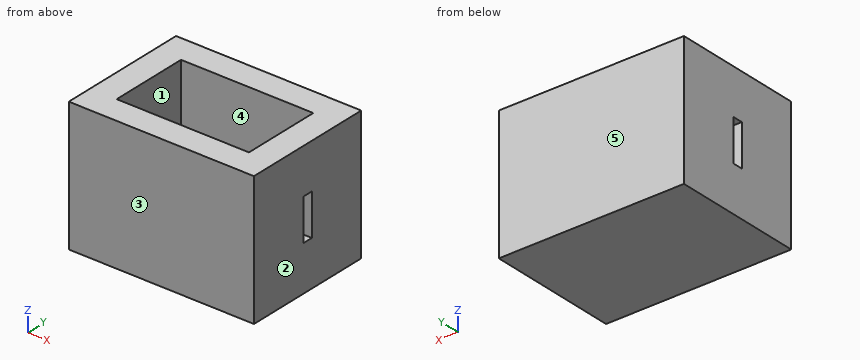
```python
from build123d import *

# Parameters (mm, degrees)
IZIM1_W                     = 12.7
IZIM1_H                     = 12.7
Y_KSEKLIK_EKSTR_ZYON1_DEPTH = 2.54
IZIM2_W                     = 4
IZIM2_H                     = 1
KES_EKSTR_ZYON1_DEPTH       = 2.54
IZIM3_W                     = 12.7
IZIM3_H                     = 12.7
Y_KSEKLIK_EKSTR_ZYON2_DEPTH = 2.54
IZIM4_W                     = 12.7
IZIM4_H                     = 12.7
Y_KSEKLIK_EKSTR_ZYON3_DEPTH = 2.54
IZIM5_W                     = 12.7
IZIM5_H                     = 7.62
Y_KSEKLIK_EKSTR_ZYON4_DEPTH = 2.54
IZIM7_W                     = 12.7
IZIM7_H                     = 12.7
Y_KSEKLIK_EKSTR_ZYON6_DEPTH = 2.54
IZIM8_W                     = 4
IZIM8_H                     = 1
KES_EKSTR_ZYON2_DEPTH       = 2.54


with BuildPart() as part:
    # Çizim1 → Yükseklik-Ekstrüzyon1 (new body)
    with BuildSketch(Plane(origin=(0, 0, 0), x_dir=(0, 0, -1), z_dir=(1, 0, 0))):
        Rectangle(IZIM1_W, IZIM1_H)
    extrude(amount=Y_KSEKLIK_EKSTR_ZYON1_DEPTH)

    # Çizim2 → Kes-Ekstrüzyon1 (cut)
    with BuildSketch(Plane(origin=(2.54, 0, 0), x_dir=(0, 0, -1), z_dir=(1, 0, 0))):
        Rectangle(IZIM2_W, IZIM2_H)
    extrude(amount=-KES_EKSTR_ZYON1_DEPTH, mode=Mode.SUBTRACT)

    # Çizim3 → Yükseklik-Ekstrüzyon2 (add)
    with BuildSketch(Plane(origin=(0, 6.35, 0), x_dir=(1, 0, 0), z_dir=(0, 1, 0))):
        with Locations((8.89, 0)):
            Rectangle(IZIM3_W, IZIM3_H)
    extrude(amount=-Y_KSEKLIK_EKSTR_ZYON2_DEPTH)

    # Çizim4 → Yükseklik-Ekstrüzyon3 (add)
    with BuildSketch(Plane.XZ.offset(6.35)):
        with Locations((8.89, 0)):
            Rectangle(IZIM4_W, IZIM4_H)
    extrude(amount=-Y_KSEKLIK_EKSTR_ZYON3_DEPTH)

    # Çizim5 → Yükseklik-Ekstrüzyon4 (add)
    with BuildSketch(Plane(origin=(0, 0, -6.35), x_dir=(-1, 0, 0), z_dir=(0, 0, -1))):
        with Locations((-8.89, 0)):
            Rectangle(IZIM5_W, IZIM5_H)
    extrude(amount=-Y_KSEKLIK_EKSTR_ZYON4_DEPTH)

    # Çizim7 → Yükseklik-Ekstrüzyon6 (add)
    with BuildSketch(Plane(origin=(15.24, 0, 0), x_dir=(0, 0, -1), z_dir=(1, 0, 0))):
        Rectangle(IZIM7_W, IZIM7_H)
    extrude(amount=Y_KSEKLIK_EKSTR_ZYON6_DEPTH)

    # Çizim8 → Kes-Ekstrüzyon2 (cut)
    with BuildSketch(Plane.ZY.offset(-15.24)):
        Rectangle(IZIM8_W, IZIM8_H)
    extrude(amount=-KES_EKSTR_ZYON2_DEPTH, mode=Mode.SUBTRACT)


solid = part.part
```
Geometry: final body of the model. Coordinates: model frame, mm. Face numbers are marked on the shaded views. A direction names the side the tool comes from. Round coordinates to 2 decimals unless told otherwise and drop trailing zeros. Order: outer loops, then holes, each group sorted by start corner. A loop starts at its lowest first (then second) coordinate and runs counter-clockwise, first axis right, second up. Notation, with made-up numbers: (45.5, 69) -> (56.5, 69) arc R21 ccw to (56.5, 106) -> close; hole circle Ø11 at (-40, 23.5). An arc over 180 degrees is marked (long way). Use one line per item in the form item = value. Start each with the question number.
1. Draft query along Y for the marked faces 1, 2 and 3. Return one class per face: pulls with the +Y half, pulls with the -Y half, needs draft (parallel to the pull), parting line crosses it, or undercut.
2. Pin query (flat end, axial travel): pin 1 Ø6 at (x, y) = (7.5, 0.5) entering from +Z. Return the tip coordinate at first contact, or that it passes through.
3. Cut plane D-D (x = 5.5). Return the cut outline in (y, z), then the cut area to 3 significant figures.
4. Reachability of the marked faces 4 and 5 from +Z, -Z, +X, -X, +Y, -Y: full face, straight path, thin tool, end or side. Return the list, or none.
5. Cut plane B-B (z = 2.5). Return the cut outline in (x, y).
6. Cut plane A-A (z = 1). Return the cut outline in (x, y).
7. Line query: probe 1 along Y at (x, z) = (6.75, 0); probe 2 along X at (y, z) = (1.75, -3.25); probe 3 along Y at (x, z) = (15.5, -1). Output: solid intervals per line, ascending.
8. Cut plane C-C (y = 2). Return the cut outline in (x, z).
Solution:
q1.face_1 = undercut
q1.face_2 = needs draft
q1.face_3 = pulls with the -Y half
q2.pin_1 = -3.81
q3.outline = (-6.35, -6.35) -> (6.35, -6.35) -> (6.35, 6.35) -> (3.81, 6.35) -> (3.81, -3.81) -> (-3.81, -3.81) -> (-3.81, 6.35) -> (-6.35, 6.35) -> close
q3.area = 83.9 mm^2
q4.face_4 = +Z
q4.face_5 = +Z, -Z, +X, -X, +Y
q5.outline = (0, -6.35) -> (17.78, -6.35) -> (17.78, 6.35) -> (0, 6.35) -> close; hole (2.54, -3.81) -> (15.24, -3.81) -> (15.24, 3.81) -> (2.54, 3.81) -> close
q6.outline = (0, -6.35) -> (17.78, -6.35) -> (17.78, -0.5) -> (15.24, -0.5) -> (15.24, -3.81) -> (2.54, -3.81) -> (2.54, -0.5) -> (0, -0.5) -> close; (0, 0.5) -> (2.54, 0.5) -> (2.54, 3.81) -> (15.24, 3.81) -> (15.24, 0.5) -> (17.78, 0.5) -> (17.78, 6.35) -> (0, 6.35) -> close
q7.probe_1 = -6.35 to -3.81, 3.81 to 6.35
q7.probe_2 = 0 to 2.54, 15.24 to 17.78
q7.probe_3 = -6.35 to -0.5, 0.5 to 6.35
q8.outline = (0, -6.35) -> (17.78, -6.35) -> (17.78, 6.35) -> (15.24, 6.35) -> (15.24, -3.81) -> (2.54, -3.81) -> (2.54, 6.35) -> (0, 6.35) -> close
